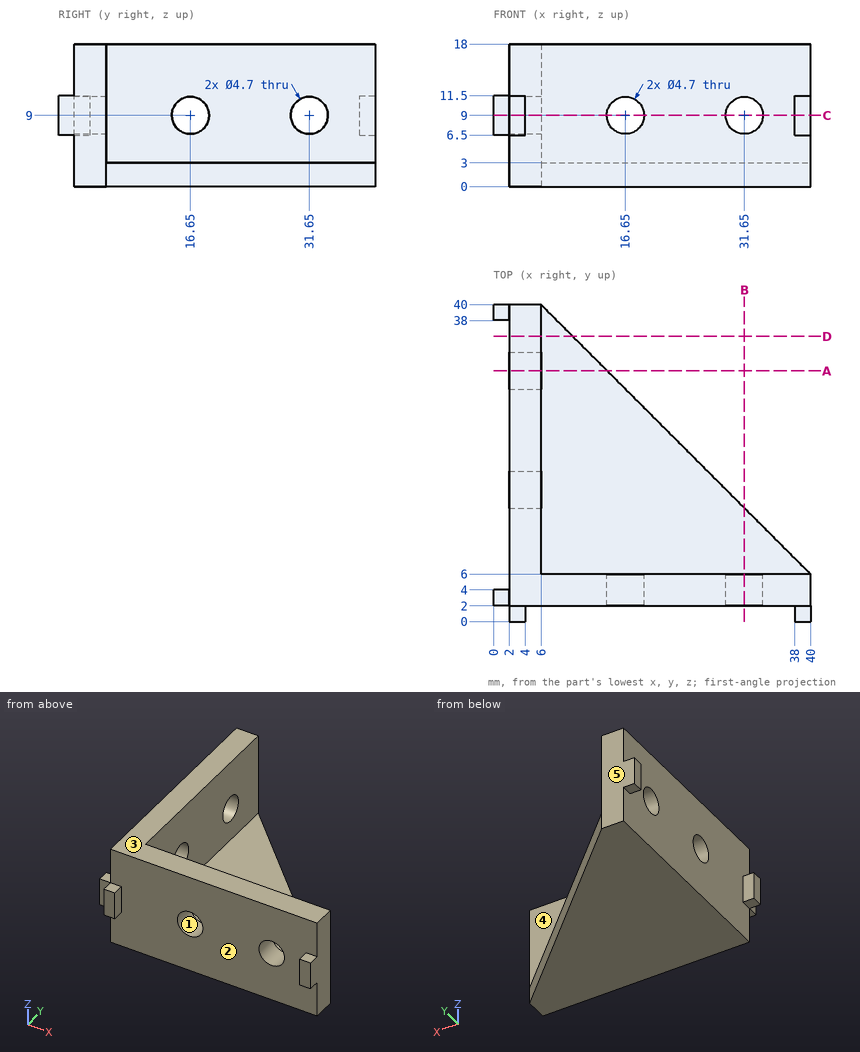
Check sheet for the drawn part. Datum: minimum x, y, z corner. Units: mm. A direction names the side the tool comes from. Round coordinates to 2 decimals unless told otherwise and drop trailing zeros. Write each loop counter-clockwise with the first axis right and the second up, starting at its lowest first coordinate (ties: lowest second). Pieces come first, ordered by that corner, then holes. Notation, with made-up numbers: (84.5, 66) - (117.5, 66) arc R22 cw to (117.5, 89) - close; hole circle Ø11 at (38.25, 35.5). An arc over 180 degrees is marked (long way). Return JSON: item names as keys, results as strings.
Q1. Draft check along Z on the marked faces 1, 2 and 3. Enter one of: released by +Z, released by -Z, zero draft, split by the parting line, or undercut.
Returned:
{"face 1": "undercut", "face 2": "zero draft", "face 3": "released by +Z"}
Q2. Depth check by flat-ended pin: P1, Ø5.5, axis at y = 13, z = 11.5, coming from the -X side; P2, Ø1, axis at x = 1, y = 3.5, coming from the -Z side; P3, Ø2, axis at x = 9, z = 10.5, coming from the -Y side. Enter the tip coordinate at first touch or a pass-through.
Returned:
{"P1": "stops at x = 2", "P2": "stops at z = 6.5", "P3": "stops at y = 2"}
Q3. Access from +Z, -Z, +X, -X, +Y, -Y to the whole of each face (thin tool, end or side, straight path). Record for the marked faces 4 and 5.
Returned:
{"face 4": "+Z, +X, +Y", "face 5": "+Z, -Z, +X, -X, +Y"}
Q4. Scan lines: L1, parallel to X at y = 4.5, z = 9; L2, parallel to X at y = 3.4, z = 9. Record each from-to range of solid material in increasing order. Write a range as from..to.
Returned:
{"L1": "x = 2..14.3, 19..29.3, 34..40", "L2": "x = 0..14.3, 19..29.3, 34..40"}
Q5. Cross-section at C-C (z = 9). Give the number of separate pieces and of enclosed holes in the cut face, then the cut area to 3 significant figures.
Returned:
{"separate pieces": "5", "enclosed holes": "0", "area": "229 mm²"}
Q6. Cross-section at D-D (y = 36). Record the boundary of the cut face in (x, z), then the cut area to 3 significant figures.
Returned:
{"outline": "(2, 0) - (10, 0) - (10, 3) - (6, 3) - (6, 18) - (2, 18) - close", "area": "84.0 mm²"}
Q7. Cross-section at A-A (y = 31.65). Record the boundary of the cut face in (x, z).
Returned:
{"outline": "(2, 0) - (14.35, 0) - (14.35, 3) - (6, 3) - (6, 6.65) - (2, 6.65) - close; (2, 11.35) - (6, 11.35) - (6, 18) - (2, 18) - close"}
